Check sheet for the modelled part. Datum: model origin and axes. Units: mm. Face numbers are marked on the shaded views. A direction names the side the tool comes from. Round coordinates to 2 decimals unless told otherwise and drop trailing zeros. Order: outer loops, then holes, each group sorted by start corner. A loop starts at its lowest first (then second) coordinate and runs counter-clockwise, first axis right, second up.
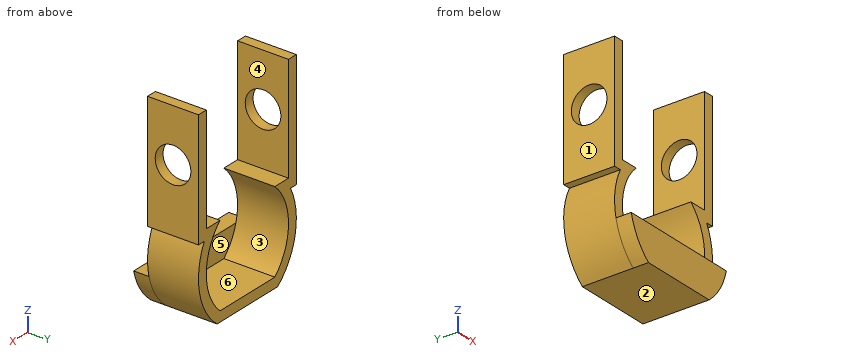
```python
from build123d import *

# Parameters (mm, degrees)
BOSS_EXTRUDE1_DEPTH = 10
SKETCH2_R           = 3.5
CUT_EXTRUDE1_DEPTH  = 26
BOSS_EXTRUDE2_DEPTH = 3


with BuildPart() as part:
    # Sketch1 → Boss-Extrude1 (new body)
    with BuildSketch(Plane(origin=(0, 0, 0), x_dir=(1, 0, 0), z_dir=(0, 1, 0))):
        with BuildLine():
            Line((7, 16), (-7, 16))
            ThreePointArc((-7, 16), (-10.5, 8), (-7, 0))
            Line((-7, 0), (-10.5, 0))
            Line((-10.5, 0), (-10.5, -21))
            Line((-10.5, -21), (-12.5, -21))
            Line((-12.5, -21), (-12.5, 2))
            Line((-12.5, 2), (-11.018793277, 2))
            ThreePointArc((-11.018793277, 2), (-12.238312239, 10.584439081), (-7.745064294, 18))
            Line((-7.745064294, 18), (7.745064294, 18))
            ThreePointArc((7.745064294, 18), (12.238312239, 10.584439081), (11.018793277, 2))
            Line((11.018793277, 2), (12.5, 2))
            Line((12.5, 2), (12.5, -21))
            Line((12.5, -21), (10.5, -21))
            Line((10.5, -21), (10.5, 0))
            Line((10.5, 0), (7, 0))
            ThreePointArc((7, 0), (10.5, 8), (7, 16))
        make_face()
    extrude(amount=BOSS_EXTRUDE1_DEPTH)

    # Sketch2 → Cut-Extrude1 (cut, through all)
    with BuildSketch(Plane.ZY.offset(12.5)):
        with Locations((10.5, 5)):
            Circle(SKETCH2_R)
    extrude(amount=-CUT_EXTRUDE1_DEPTH, mode=Mode.SUBTRACT)

    # Sketch3 → Boss-Extrude2 (add)
    with BuildSketch(Plane.XZ):
        with BuildLine():
            Line((-12.146112723, -11), (12.146112723, -11))
            ThreePointArc((12.146112723, -11), (10.521970317, -14.862383465), (7.745064294, -18))
            Line((7.745064294, -18), (-7.745064294, -18))
            ThreePointArc((-7.745064294, -18), (-10.521970317, -14.862383465), (-12.146112723, -11))
        make_face()
    extrude(amount=BOSS_EXTRUDE2_DEPTH)


solid = part.part
```
Item 1: Sectioned sample at B-B (y = 5). Record the cut outline in (x, z), and give its area (3 significant figures).
Answer:
outline: (-12.5, -2) - (-11.02, -2) arc R12.89 ccw to (-7.75, -18) - (7.75, -18) arc R12.89 ccw to (11.02, -2) - (12.5, -2) - (12.5, 7) - (10.5, 7) - (10.5, 0) - (7, 0) arc R10.89 cw to (7, -16) - (-7, -16) arc R10.89 cw to (-7, 0) - (-10.5, 0) - (-10.5, 7) - (-12.5, 7) - close; (-12.5, 14) - (-10.5, 14) - (-10.5, 21) - (-12.5, 21) - close; (10.5, 14) - (12.5, 14) - (12.5, 21) - (10.5, 21) - close
area: 170 mm2
Item 2: Sectioned sample at D-D (x = -2.75). Record the cut outline in (y, z).
Answer:
outline: (-3, -18) - (10, -18) - (10, -16) - (0, -16) - (0, -11) - (-3, -11) - close
Item 3: Scan lines: line 1 along Y through (x, z) = (-11.05, 10.5); line 2 along X through (y, z) = (9, 10); line 3 along Z through (x, y) = (-2.25, 1). Record each from-to range of solid material in increasing order.
Answer:
line 1: y = 0 to 1.5, 8.5 to 10
line 2: x = -12.5 to -10.5, 10.5 to 12.5
line 3: z = -18 to -16
Item 4: Go/stop test with flat-tipped pins: P1, Ø2.5, axis at x = 0, z = -13, coming from the +Y side; P2, Ø2, axis at y = -1.5, z = 12.5, coming from the -X side; P3, Ø3, axis at x = 2.5, y = 6.5, coming from the +Z side; P4, Ø3, axis at x = -8, y = 7, coming from the +Z side. Record where each tip stops, or that it passes through.
Answer:
P1: stops at y = 0
P2: passes through
P3: stops at z = -16
P4: stops at z = 0
Item 5: Access from +Z, -Z, +X, -X, +Y, -Y to the whole of each face (thin tool, end or side, straight path). Record for the marked faces 4, 5 and 6.
Answer:
face 4: +Z, +Y, -Y
face 5: +Y
face 6: +Z, +Y
Item 6: Sectioned sample at C-C (z = 10.5). Record the cut outline in (x, y), and give its area (3 significant figures).
Answer:
outline: (-12.5, 0) - (-10.5, 0) - (-10.5, 1.5) - (-12.5, 1.5) - close; (-12.5, 8.5) - (-10.5, 8.5) - (-10.5, 10) - (-12.5, 10) - close; (10.5, 0) - (12.5, 0) - (12.5, 1.5) - (10.5, 1.5) - close; (10.5, 8.5) - (12.5, 8.5) - (12.5, 10) - (10.5, 10) - close
area: 12.0 mm2
Item 7: Release check for a two-part mould opening along Z. For the marked faces 1, 2 and 3 record: released by +Z, released by -Z, zero draft, split by the parting line, or undercut.
Answer:
face 1: zero draft
face 2: released by -Z
face 3: undercut
Item 8: Sectioned sample at A-A (z = 5). Record the cut outline in (x, y).
Answer:
outline: (-12.5, 0) - (-10.5, 0) - (-10.5, 10) - (-12.5, 10) - close; (10.5, 0) - (12.5, 0) - (12.5, 10) - (10.5, 10) - close
